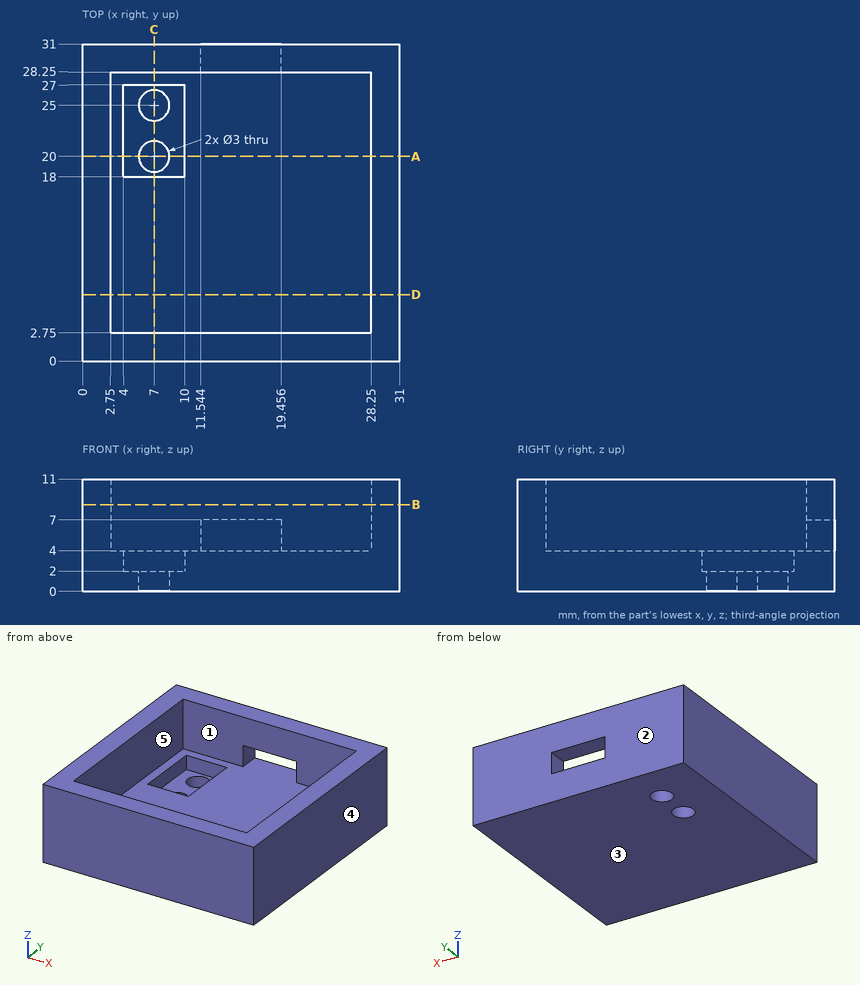
Source: three-view drawing plus pictorial views. Frame: mm from the lowest corner of the part. A direction names the side the tool comes from. Give positions to 0.01 mm unless a question says otherwise; leave off trailing zeros. Order: outer loops, then holes, each group sorted by start corner. A loop starts at its lowest first (then second) coordinate and runs counter-clockwise, first axis right, second up. Notation, with made-up numbers: (60.5, -21.5) -> (82.5, -21.5) arc R22 cw to (82.5, 11.5) -> close; hole circle Ø6 at (-9, 6.5). An arc over 180 degrees is marked (long way). Write each question's results on one line, items separated by ' | '. Start each with the question number.
Item 1: Cut plane B-B on z = 8.5. Return the cut outline in (x, y).
Item 2: Line query: line 1 (Y direction, x = 7, z = 1.5); line 2 (X direction, y = 16, z = 6.75). Output: solid intervals per line, ascending.
Item 3: Mould query, pull axis Y, two halves, no side actions, for the marked faces 1, 2 and 3. Classes: pulls with the +Y half, pulls with the -Y half, needs draft (parallel to the pull), parting line crosses it, or undercut.
Item 4: Contact query for flat-ended pins moving along their axis: P1, Ø7.5, axis at x = 17, y = 18, coming from the +Z side; P2, Ø3, axis at x = 6, y = 20.5, coming from the +Z side. Output: stop coordinate, or through.
Item 5: Cut plane C-C on x = 7. Return the cut outline in (y, z).
Item 6: Cut plane D-D on y = 6.5. Return the cut outline in (x, z).
Item 7: Set-up query: the marked faces 4 and 5. Return all of +Z, -Z, +X, -X, +Y, -Y with unobstructed straight access to the full face (end or side cutting, diameter ignored); none if empty.
Item 8: Cut plane A-A on y = 20. Return the cut outline in (x, z).
Established:
1) outline: (0, 0) -> (31, 0) -> (31, 31) -> (0, 31) -> close; hole (2.75, 2.75) -> (28.25, 2.75) -> (28.25, 28.25) -> (2.75, 28.25) -> close
2) line 1: 0 to 18.5, 21.5 to 23.5, 26.5 to 31 | line 2: 0 to 2.75, 28.25 to 31
3) face 1: undercut | face 2: pulls with the +Y half | face 3: needs draft
4) P1: z = 4 | P2: z = 2
5) outline: (0, 0) -> (18.5, 0) -> (18.5, 2) -> (18, 2) -> (18, 4) -> (2.75, 4) -> (2.75, 11) -> (0, 11) -> close; (21.5, 0) -> (23.5, 0) -> (23.5, 2) -> (21.5, 2) -> close; (26.5, 0) -> (31, 0) -> (31, 11) -> (28.25, 11) -> (28.25, 4) -> (27, 4) -> (27, 2) -> (26.5, 2) -> close
6) outline: (0, 0) -> (31, 0) -> (31, 11) -> (28.25, 11) -> (28.25, 4) -> (2.75, 4) -> (2.75, 11) -> (0, 11) -> close
7) face 4: +Z, -Z, +X, +Y, -Y | face 5: +Z
8) outline: (0, 0) -> (5.5, 0) -> (5.5, 2) -> (4, 2) -> (4, 4) -> (2.75, 4) -> (2.75, 11) -> (0, 11) -> close; (8.5, 0) -> (31, 0) -> (31, 11) -> (28.25, 11) -> (28.25, 4) -> (10, 4) -> (10, 2) -> (8.5, 2) -> close
